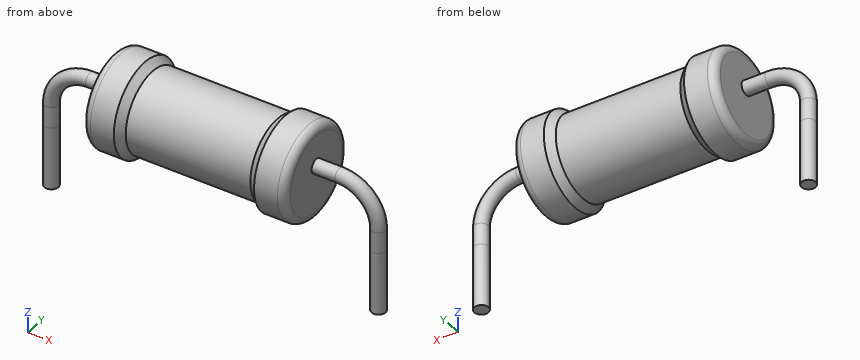
```python
from build123d import *

# Parameters (mm, degrees)
SKETCH_1_R      = 0.45
FILLET_1_R      = 0.5
SKETCH_4_R      = 0.45
EXTRUDE_1_DEPTH = 4


with BuildPart() as part:
    # Эскиз2 → Повернуть1 (revolve)
    with BuildSketch(Plane.XY.offset(3.35), mode=Mode.PRIVATE) as revolve_1_sk:
        Polygon((4, 0), (17, 0), (17, 3), (15, 3), (14.5, 2.6), (6.5, 2.6), (6, 3), (4, 3), align=None)
    revolve(revolve_1_sk.sketch.rotate(Axis((0, 0, 3.35), (1, 0, 0)), 90), axis=Axis((0, 0, 3.35), (1, 0, 0)))

    # По траектории1: sweep along a path in Эскиз3
    with BuildLine(Plane(origin=(0, 0, 0), x_dir=(1, 0, 0), z_dir=(0, 1, 0))) as sweep_1_path:
        Line((20.5, 0), (20.5, -1.35))
        ThreePointArc((20.5, -1.35), (19.914213562, -2.764213562), (18.5, -3.35))
        Line((18.5, -3.35), (2.5, -3.35))
        ThreePointArc((2.5, -3.35), (1.085786438, -2.764213562), (0.5, -1.35))
        Line((0.5, -1.35), (0.5, 0))
    # Эскиз1 → По траектории1 (sweep)
    with BuildSketch(Plane.XY):
        Circle(SKETCH_1_R)
    sweep(path=sweep_1_path.line)

    # Скругление1
    fillet_1_edges = [part.edges().sort_by_distance(p)[0] for p in [
        (17, 0, 0.35),
        (4, 0, 0.35),
    ]]
    fillet(fillet_1_edges, radius=FILLET_1_R)

    # Эскиз4 → Вытянуть1 (add)
    with BuildSketch(Plane(origin=(0, 0, 0), x_dir=(-1, 0, 0), z_dir=(0, 0, -1))):
        Circle(SKETCH_4_R)
        with Locations((-21, 0)):
            Circle(SKETCH_4_R)
    extrude(amount=EXTRUDE_1_DEPTH)


solid = part.part
```
Source: CAD feature listing. Evaluate the final solid. Frame: model axes, mm. Round coordinates to 2 decimals unless told otherwise and drop trailing zeros. Loops run counter-clockwise (first coordinate to the right, second up) from the corner with the lowest first, then second, coordinate; pieces in that order, holes last.
(1) Contact query for flat-ended pins moving along their axis: pin 1 Ø3 at (x, y) = (11.5, 2) entering from -Z; pin 2 Ø1 at (x, y) = (12, -1.5) entering from -Z; pin 3 Ø1.5 at (y, z) = (1, 2.5) entering from +X. Output: stop coordinate, or through.
From the geometry:
pin 1: stops at z = 0.8
pin 2: stops at z = 0.95
pin 3: stops at x = 21.2
(2) Section query B-B (z = -1.5). Output: boundary loops of the cut face in (x, y).
From the geometry:
outline: circle Ø0.9 at (0, 0); circle Ø0.9 at (21, 0)
(3) Section query D-D (z = 1.75). Give the number of separate pieces and of enclosed holes in the cut face, and give its area (3 significant figures).
From the geometry:
separate pieces: 3
enclosed holes: 0
area: 58.7 mm2
(4) Section query C-C (x = 14.75). Output: boundary loops of the cut face in (y, z).
From the geometry:
outline: circle Ø5.6 at (0, 3.35)
(5) Material intervals for probe 1 along X at (y, z) = (-1, 4.5); probe 2 along X at (y, z) = (0.1, 2.5); probe 3 along X at (y, z) = (-1.7, 1.25), sorted ascending.
From the geometry:
probe 1: x = 4 to 17
probe 2: x = -0.2 to 0.79, 4 to 17, 20.21 to 21.2
probe 3: x = 4.04 to 6.37, 14.63 to 16.96
